Can you work these out from the model? Positions are in its coordinate system, mm. Face numbers are marked on the shaded views. Round coordinates to 2 decimals unless told otherwise and drop trailing zeros. Loops run counter-clockwise (first coordinate to the right, second up) from the corner with the lowest first, then second, coordinate; pieces in that order, holes last.
```python
from build123d import *

# Parameters (mm, degrees)
F0_R     = 3
F1_DEPTH = 3.95
F0_R_2   = 2.499
F2_DEPTH = 3.45
F3_R     = 3.69999
F4_R     = 3.69999


# Not quite as in the source:
# - a fillet or chamfer is up to 0.001 mm smaller than in the source, because OpenCascade refuses the exact size


with BuildPart() as f1:
    # F0 (on Front) → F1 (new body, symmetric)
    with BuildSketch(Plane.XZ):
        Polygon((-43.5, 0), (0, 0), (43.5, 0), (43.5, 7.4), (-43.5, 7.4), align=None)
        with Locations((-40, 3.7)):
            Circle(F0_R, mode=Mode.SUBTRACT)
        with Locations((-32, 3.7)):
            Circle(F0_R, mode=Mode.SUBTRACT)
        with Locations((-24, 3.7)):
            Circle(F0_R, mode=Mode.SUBTRACT)
        with Locations((-16, 3.7)):
            Circle(F0_R, mode=Mode.SUBTRACT)
        with Locations((-8, 3.7)):
            Circle(F0_R, mode=Mode.SUBTRACT)
        with Locations((0, 3.7)):
            Circle(F0_R, mode=Mode.SUBTRACT)
        with Locations((8, 3.7)):
            Circle(F0_R, mode=Mode.SUBTRACT)
        with Locations((16, 3.7)):
            Circle(F0_R, mode=Mode.SUBTRACT)
        with Locations((24, 3.7)):
            Circle(F0_R, mode=Mode.SUBTRACT)
        with Locations((32, 3.7)):
            Circle(F0_R, mode=Mode.SUBTRACT)
        with Locations((40, 3.7)):
            Circle(F0_R, mode=Mode.SUBTRACT)
    extrude(amount=F1_DEPTH, both=True)

    # F0 (on Front) → F2 (join, symmetric)
    with BuildSketch(Plane.XZ):
        with Locations((-40, 3.7)):
            Circle(F0_R)
        with Locations((-40, 3.7)):
            Circle(F0_R_2, mode=Mode.SUBTRACT)
        with Locations((-32, 3.7)):
            Circle(F0_R)
        with Locations((-32, 3.7)):
            Circle(F0_R_2, mode=Mode.SUBTRACT)
        with Locations((-24, 3.7)):
            Circle(F0_R)
        with Locations((-24, 3.7)):
            Circle(F0_R_2, mode=Mode.SUBTRACT)
        with Locations((-16, 3.7)):
            Circle(F0_R)
        with Locations((-16, 3.7)):
            Circle(F0_R_2, mode=Mode.SUBTRACT)
        with Locations((-8, 3.7)):
            Circle(F0_R)
        with Locations((-8, 3.7)):
            Circle(F0_R_2, mode=Mode.SUBTRACT)
        with Locations((0, 3.7)):
            Circle(F0_R)
        with Locations((0, 3.7)):
            Circle(F0_R_2, mode=Mode.SUBTRACT)
        with Locations((8, 3.7)):
            Circle(F0_R)
        with Locations((8, 3.7)):
            Circle(F0_R_2, mode=Mode.SUBTRACT)
        with Locations((16, 3.7)):
            Circle(F0_R)
        with Locations((16, 3.7)):
            Circle(F0_R_2, mode=Mode.SUBTRACT)
        with Locations((24, 3.7)):
            Circle(F0_R)
        with Locations((24, 3.7)):
            Circle(F0_R_2, mode=Mode.SUBTRACT)
        with Locations((32, 3.7)):
            Circle(F0_R)
        with Locations((32, 3.7)):
            Circle(F0_R_2, mode=Mode.SUBTRACT)
        with Locations((40, 3.7)):
            Circle(F0_R)
        with Locations((40, 3.7)):
            Circle(F0_R_2, mode=Mode.SUBTRACT)
    extrude(amount=F2_DEPTH, both=True)

    # F3 (radius 3.7 in the source; OpenCascade refuses exactly that, so slightly less here)
    f3_edges = [f1.edges().sort_by_distance(p)[0] for p in [
        (-43.5, 0, 7.4),
        (-43.5, 0, 0),
    ]]
    fillet(f3_edges, radius=F3_R)

    # F4 (radius 3.7 in the source; OpenCascade refuses exactly that, so slightly less here)
    f4_edges = [f1.edges().sort_by_distance(p)[0] for p in [
        (43.5, 0, 7.4),
        (43.5, 0, 0),
    ]]
    fillet(f4_edges, radius=F4_R)


solid = f1.part
```
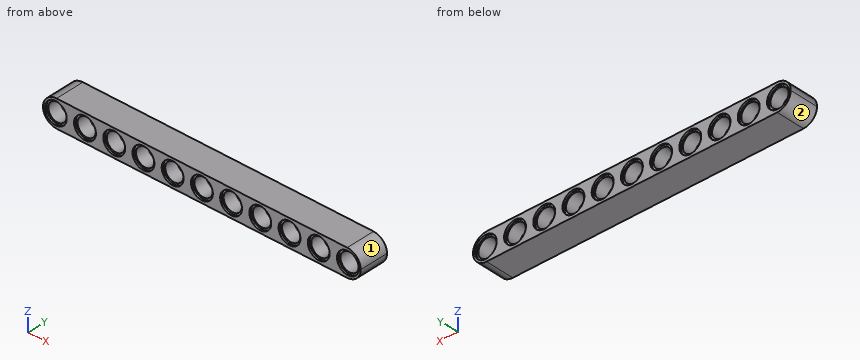
(1) We'd pull the mould along Z, two halves only. Please class the marked faces 1 and 2: released by +Z, released by -Z, zero draft, split by the parting line, or undercut.
(2) If I drill on line 1 (Z direction, x = 32, y = -1.25); line 2 (Z direction, x = 24, y = 3.7); line 3 (Y direction, x = -10.5, z = 5.25), over which ranges is the centre line in solid material (lowest first)?
(3) Suppose I cut it at B-B (y = 1.75). Give the number of separate pieces and of enclosed holes in the cut face, then the cut area to 3 significant figures.
(4) For pin 1 (1.8 mm diameter, centred on x = -17, z = 5, fed in from -Y), with a flat end and sliding along its axis, tell me the tip position at first contact or that it passes through.
(5) Suppose I cut it at A-A (x = -16). Write out the boundary of the cut face in (y, z), then the cut area to 3 significant figures.
Check result:
1. face 1: released by +Z
1. face 2: released by -Z
2. line 1: z = 0 to 1.2, 6.2 to 7.4
2. line 2: z = 0 to 0.7, 6.7 to 7.4
2. line 3: y = -3.45 to 3.45
3. separate pieces: 1
3. enclosed holes: 11
3. area: 416 mm2
4. pin 1: stops at y = -3.45
5. outline: (-3.95, 0) - (3.95, 0) - (3.95, 0.7) - (3.45, 0.7) - (3.45, 1.2) - (-3.45, 1.2) - (-3.45, 0.7) - (-3.95, 0.7) - close; (-3.95, 6.7) - (-3.45, 6.7) - (-3.45, 6.2) - (3.45, 6.2) - (3.45, 6.7) - (3.95, 6.7) - (3.95, 7.4) - (-3.95, 7.4) - close
5. area: 18.0 mm2
